Design review of the part shown in the three views and the two pictorial views. Dimensions are in mm from the part's minimum x, y and z. Coordinates: 2 decimals unless noted, no trailing zeros. Order: outer loops, then holes, each group sorted by start corner. A loop starts at its lowest first (then second) coordinate and runs counter-clockwise, first axis right, second up. Notation, with made-up numbers: (81.5, 8) -> (86.5, 8) arc R29 ccw to (86.5, 42) -> close; hole circle Ø4 at (-25.75, 76). An arc over 180 degrees is marked (long way). Answer as a JSON object with one key per item and string values. Group by question number.
1) Add section C-C, the plane x = 49. Write out the cut boundary in (y, z), then the cut area to 3 significant figures.
2) Add section B-B, the plane y = 34. Write out the cut boundary in (x, z), then the cut area to 3 significant figures.
3) Draft analysis for pull direction X (two halves, no side actions). For the marked faces 1 and 2, state which applies: +X half, -X half, draft (parallel to the pull), parting line (faces both ways), or undercut.
4) Add section A-A, the plane z = 2.4. Write out the cut boundary in (x, y).
5) For pin 1 (2 mm diameter, centred on y = 17.5, z = 3.5, fed in from -X); pin 2 (1.5 mm diameter, centred on x = 45, z = 2.5, fed in from +Y); pin 3 (6 mm diameter, centred on x = 46.5, y = 43, fed in from +Z), all flat-tipped, find the tip position at first contact; note any pin that passes through.
6) Wall thickness on L1, parallel to Z at x = 32.5, y = 12; L2, parallel to X at y = 11.5, z = 3.15; L3, parallel to X at y = 41, z = 1.5: over which ranges is each line inside the solid? List them lowest first.
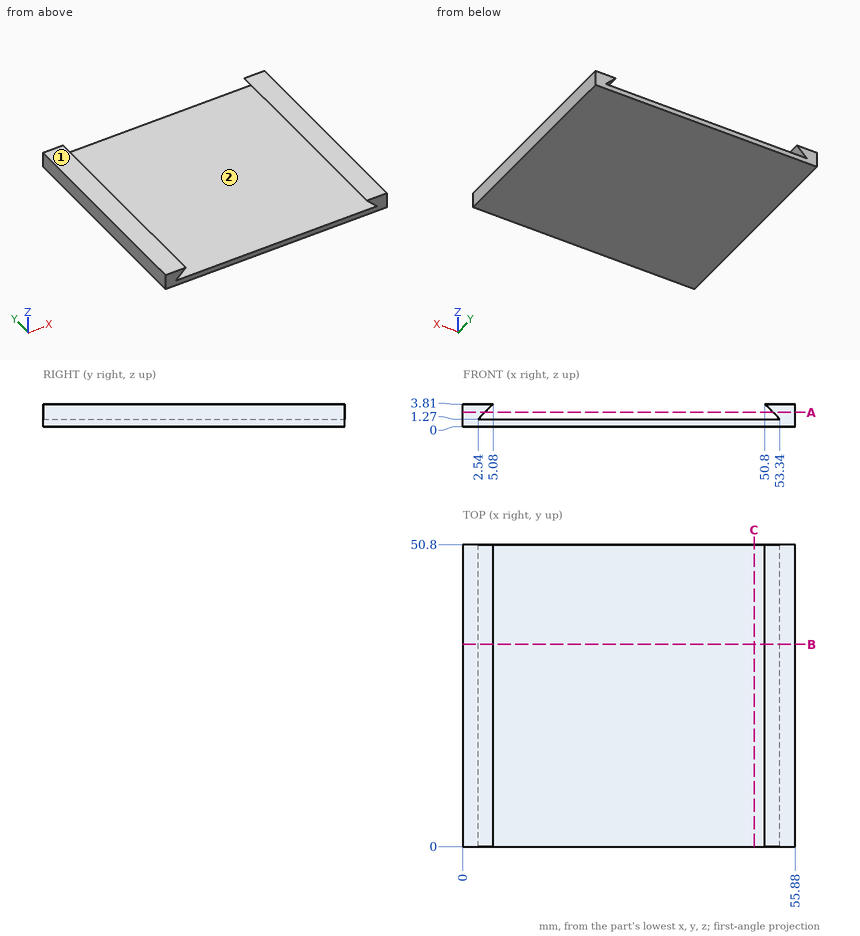
Output values:
{
 "1": {"outline": "(0, 0) -> (50.8, 0) -> (50.8, 1.27) -> (0, 1.27) -> close", "area": "64.5 mm²"},
 "2": {"outline": "(0, 0) -> (55.88, 0) -> (55.88, 3.81) -> (50.8, 3.81) -> (53.34, 1.27) -> (2.54, 1.27) -> (5.08, 3.81) -> (0, 3.81) -> close", "area": "90.3 mm²"},
 "3": {"face 1": "draft", "face 2": "undercut"},
 "4": {"outline": "(0, 0) -> (3.67, 0) -> (3.67, 50.8) -> (0, 50.8) -> close; (52.21, 0) -> (55.88, 0) -> (55.88, 50.8) -> (52.21, 50.8) -> close"},
 "5": {"pin 1": "stops at x = 0", "pin 2": "passes through", "pin 3": "stops at z = 1.27"},
 "6": {"L1": "z = 0 to 1.27", "L2": "x = 0 to 4.42, 51.46 to 55.88", "L3": "x = 0 to 2.77, 53.11 to 55.88"}
}
